Print and shaded views of the part. All mm, measured from the part's lowest x, y and z. Give positions to 0.01 mm unless a question says otherwise; leave off trailing zeros. Loops run counter-clockwise (first coordinate to the right, second up) from the corner with the lowest first, then second, coordinate; pieces in that order, holes last. Notation, with made-up numbers: (76, -13.75) - (82, -13.75) arc R18 cw to (82, 1.25) - close; hole circle Ø8 at (85.25, -32.5). An arc over 180 degrees is marked (long way). Return JSON: item names as keys, results as strings.
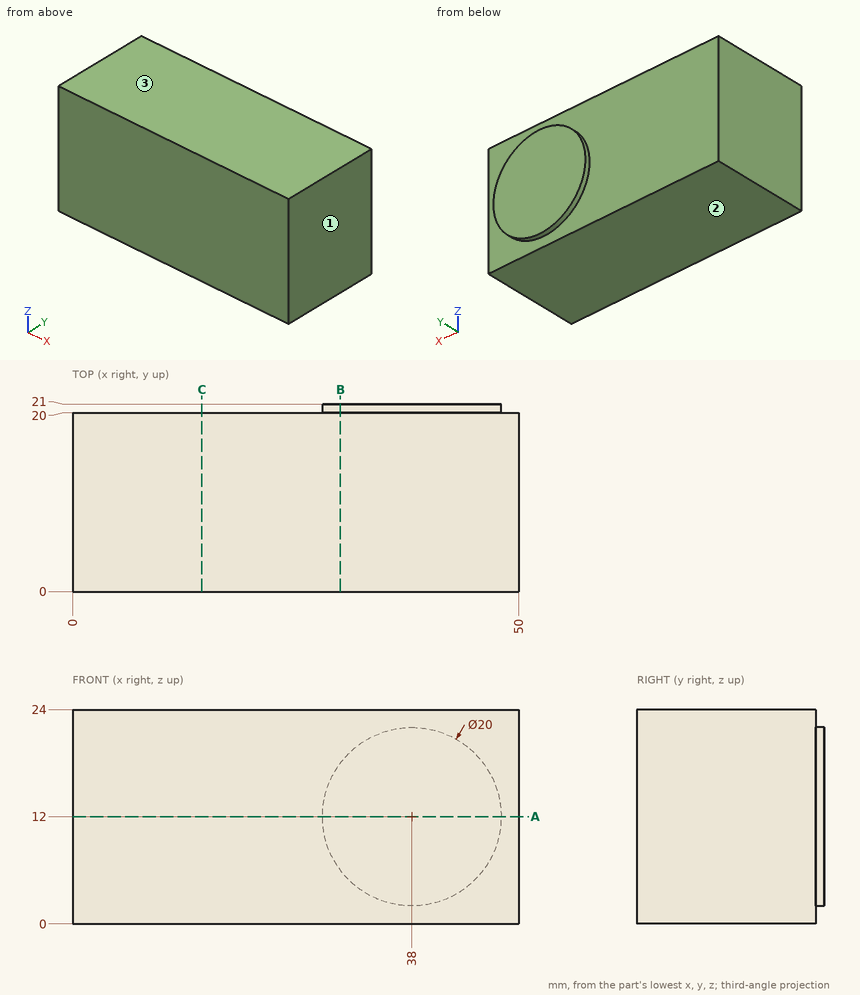
1. Cut at B-B, the plane x = 30. Write the cut outline in (y, z).
Values follow:
{"outline": "(0, 0) - (20, 0) - (20, 6) - (21, 6) - (21, 18) - (20, 18) - (20, 24) - (0, 24) - close"}
2. Cut at C-C, the plane x = 14.5. Write the cut outline in (y, z), plus the area to 3 significant figures.
Values follow:
{"outline": "(0, 0) - (20, 0) - (20, 24) - (0, 24) - close", "area": "480 mm²"}
3. Pull direction Z, two halves, no side cores. Call the marked faces 1, 2 and 3: +Z half, -Z half, draft (parallel to the pull), parting line (faces both ways), or undercut.
Values follow:
{"face 1": "draft", "face 2": "-Z half", "face 3": "+Z half"}
4. Drill centre line: probe 1 along Y at (x, z) = (11.5, 7). Where is it in solid material? Low to high.
Values follow:
{"probe 1": "y = 0 to 20"}
5. Cut at A-A, the plane z = 12. Write the cut outline in (x, y), plus the area to 3 significant figures.
Values follow:
{"outline": "(0, 0) - (50, 0) - (50, 20) - (48, 20) - (48, 21) - (28, 21) - (28, 20) - (0, 20) - close", "area": "1,020 mm²"}
